Autodesk Inventor part; units mm, degrees
ref_plane "YZ Plane" through (0, 0, 0) normal (1, 0, 0) x (0, 1, 0)
ref_plane "XZ Plane" through (0, 0, 0) normal (0, 1, 0) x (-1, 0, 0)
ref_plane "XY Plane" through (0, 0, 0) normal (0, 0, 1) x (1, 0, 0)
sketch "Sketch1" plane through (0, 0, 0) normal (0, 1, 0) x (-1, 0, 0)
  circle A0 centre (0, 0) radius 6
  line L0 (0, 0) -> (6, 0) construction
  line L1 (0, 0) -> (0, 6) construction
  circle A1 centre (15.5, 0) radius 6
  circle A2 centre (31, 0) radius 6
  circle A3 centre (0, 12) radius 6
  circle A4 centre (15.5, 12) radius 6
  circle A5 centre (31, 12) radius 6
  circle A6 centre (15.5, 0) radius 5.25
  line L2 (0, 6) -> (31, 6)
  line L3 (0, -6) -> (31, -6)
  line L4 (9.5, 12) -> (9.5, 0)
  line L5 (21.5, 12) -> (21.5, 0)
  circle A7 centre (15.5, 0) radius 4.25
  point P0 (37, 0)
  point P1 (6, 12)
  point P2 (37, 12)
  dimension "d1" = 12
  dimension "d4" = 15.5
  dimension "d7" = 12
  dimension "d10" = 10.5
  dimension "d17" = 8.5
extrude "Extrusion1" add sketch "Sketch1" along normal blind 3 contours A0 | A0 L2 L4 A1 L3 | L4 A4 L2 | L2 A1 L4 | A1 | A1 L5 L2 A2 L3 | L2 L5 A1 | A4 | A4 L5 L2 | A2 | A6 | A7
extrude "Extrusion2" add sketch "Sketch1" along normal blind 3.5 and the other way blind 1 contours A6 | A7
extrude "Extrusion3" add sketch "Sketch1" against normal blind 3.5 contours A7
sketch "Sketch2" plane through (0, 3, 0) normal (0, 1, 0) x (1, 0, 0)
  circle A0 centre (-15.5, 0) radius 5.25
  arc A1 (-21.5, -12) -> (-9.5, -12) centre (-15.5, -12) ccw
  arc A2 (0, -6) -> (0, 6) centre (0, 0) ccw
  arc A3 (-31, 6) -> (-31, -6) centre (-31, 0) ccw
  line L0 (-37, 0) -> (6, 0) construction
  line L1 (-15.5, 0) -> (-15.5, -18) construction
  point P0 (-26, 0)
  point P1 (-30, 0)
  point P2 (-34, 0)
  point P3 (-15.5, -15)
  point P4 (-15.5, -11)
  point P5 (-5, 0)
  point P6 (-1, 0)
  point P7 (3, 0)
  dimension "d20" = 11
  dimension "d22" = 15
  dimension "d23" = 10.5
  dimension "d24" = 14.5
  dimension "d25" = 18.5
hole "Hole1" at (-26, 3, 0) at (-34, 3, 0) at (-15.5, 3, 15) at (3, 3, 0) at (-5, 3, 0) direction (0, -1, 0) diameter 2 end through all
hole "Hole2" at (-30, 3, 0) at (-15.5, 3, 11) at (-1, 3, 0) direction (0, -1, 0) diameter 2.5 end through all
hole "Hole3" at (-15.5, 3.5, 0) direction (0, -1, 0) diameter 5.5 depth 1
hole "Hole4" at (-15.5, 3.5, 0) direction (0, -1, 0) diameter 3 end through all
hole "Hole5" at (-15.5, -3.5, 0) direction (0, 1, 0) diameter 6 depth 4
properties part number "servo arm BMS-630MG tripple"
Geometry: final body of the model. Coordinates: model frame, mm. A direction names the side the tool comes from. Coordinates: 2 decimals unless noted, no trailing zeros. Order: outer loops, then holes, each group sorted by start corner. A loop starts at its lowest first (then second) coordinate and runs counter-clockwise, first axis right, second up. Notation, with made-up numbers: (-2.75, 2.25) -> (52.25, 2.25) arc R8 ccw to (52.25, 8.25) -> close; hole circle Ø10 at (20.25, -2.5). An arc over 180 degrees is marked (long way). Use CSV: the item, a comma, the result in double quotes.
1) Mould query, pull axis X, two halves, no side actions, for faces 5 (the flat face through (-15, 3, 6)), 6 (the cylindrical face through (-10.255, -0.493, 0.231)), 7 (the cylindrical face through (-12.57, -1.47, 0.65)). Classes: +X half, -X half, draft (parallel to the pull), parting line (faces both ways), or undercut.
Findings:
face 5,"draft"
face 6,"parting line"
face 7,"undercut"
2) Section C-C on x = -5. Output: boundary loops of the cut face in (y, z).
Findings:
outline,"(0, -6) -> (3, -6) -> (3, -1) -> (0, -1) -> close; (0, 1) -> (3, 1) -> (3, 6) -> (0, 6) -> close"
3) Pin query (flat end, axial travel): pin 1 Ø3.5 at (x, z) = (-15.5, 0) entering from +Y; pin 2 Ø1.8 at (x, z) = (-14.5, 0) entering from -Y; pin 3 Ø5 at (x, z) = (-20.5, 15.5) entering from +Y. Return the tip coordinate at first contact, or that it passes through.
Findings:
pin 1,"stops at y = 2.5"
pin 2,"stops at y = 0.5"
pin 3,"stops at y = 3"
4) Section A-A on z = 11. Output: boundary loops of the cut face in (x, y), then the cut area to 3 significant figures.
Findings:
outline,"(-21.5, 0) -> (-16.75, 0) -> (-16.75, 3) -> (-21.5, 3) -> close; (-14.25, 0) -> (-9.5, 0) -> (-9.5, 3) -> (-14.25, 3) -> close"
area,"28.5 mm^2"
5) Access query for faces 1 (the cylindrical face through (-10.255, 3.254, 0.231)), 2 (the flat face through (-20, -1, 0)), 3 (the flat face through (-21.5, 1, 9)), 4 (the flat face through (-5, 1, 6)). Directions: +Z, -Z, +X, -X, +Y, -Y. A direction counts if a zero-diameter tool reaches every point of the face in a straight line with its end or side. Return the directions, or none.
Findings:
face 1,"+Y"
face 2,"-Y"
face 3,"+Z, -X, +Y, -Y"
face 4,"+Z, +X, +Y, -Y"
6) Section B-B on y = 1.5. State how many separate pieces and enclosed holes the cut face has, then the cut area to 3 significant figures.
Findings:
separate pieces,"1"
enclosed holes,"9"
area,"576 mm^2"
7) Line query: line 1 (Z direction, x = -15.5, y = 2.25); line 2 (Z direction, x = -1, y = 1.55); line 3 (X direction, y = 0.25, z = 7.75). Output: solid intervals per line, ascending.
Findings:
line 1,"z = -6 to -1.5, 1.5 to 9.75, 12.25 to 14, 16 to 18"
line 2,"z = -6 to -1.25, 1.25 to 6"
line 3,"x = -21.5 to -9.5"
